The model under review builds one solid part; all positions refer to its coordinate system, in mm. Face numbers are marked on the shaded views. A direction names the side the tool comes from. Round coordinates to 2 decimals unless told otherwise and drop trailing zeros. Order: outer loops, then holes, each group sorted by start corner. A loop starts at its lowest first (then second) coordinate and runs counter-clockwise, first axis right, second up.
```python
from build123d import *

# Parameters (mm, degrees)
PALMA_DEPTH   = 22
MENIQUE_DEPTH = 16
ANULAR_DEPTH  = 16
MEDIO_DEPTH   = 16
INDICE_DEPTH  = 16
PULGAR_DEPTH  = 16


with BuildPart() as part:
    # Sketch1 → Palma (new body)
    with BuildSketch(Plane.XY.offset(-11)):
        Polygon((-36, -27), (36, -27), (40, -60), (38, -118), (-38, -118), (-40, -60), align=None)
    extrude(amount=PALMA_DEPTH)

    # Sketch2 → Menique (add)
    with BuildSketch(Plane.XY.offset(-8)):
        with BuildLine():
            Line((-20.25, -112), (-20.25, -178))
            ThreePointArc((-20.25, -178), (-28.5, -186.25), (-36.75, -178))
            Line((-36.75, -178), (-36.75, -112))
            ThreePointArc((-36.75, -112), (-28.5, -103.75), (-20.25, -112))
        make_face()
    extrude(amount=MENIQUE_DEPTH)

    # Sketch3 → Anular (add)
    with BuildSketch(Plane.XY.offset(-8)):
        with BuildLine():
            Line((-1.25, -112), (-1.25, -194))
            ThreePointArc((-1.25, -194), (-9.5, -202.25), (-17.75, -194))
            Line((-17.75, -194), (-17.75, -112))
            ThreePointArc((-17.75, -112), (-9.5, -103.75), (-1.25, -112))
        make_face()
    extrude(amount=ANULAR_DEPTH)

    # Sketch4 → Medio (add)
    with BuildSketch(Plane.XY.offset(-8)):
        with BuildLine():
            Line((17.75, -112), (17.75, -202))
            ThreePointArc((17.75, -202), (9.5, -210.25), (1.25, -202))
            Line((1.25, -202), (1.25, -112))
            ThreePointArc((1.25, -112), (9.5, -103.75), (17.75, -112))
        make_face()
    extrude(amount=MEDIO_DEPTH)

    # Sketch5 → Indice (add)
    with BuildSketch(Plane.XY.offset(-8)):
        with BuildLine():
            Line((36.75, -112), (36.75, -192))
            ThreePointArc((36.75, -192), (28.5, -200.25), (20.25, -192))
            Line((20.25, -192), (20.25, -112))
            ThreePointArc((20.25, -112), (28.5, -103.75), (36.75, -112))
        make_face()
    extrude(amount=INDICE_DEPTH)

    # Sketch6 → Pulgar (add)
    with BuildSketch(Plane.XY.offset(-13)):
        with BuildLine():
            Line((43.373087285, -56.838838901), (71.373087285, -96.838838901))
            ThreePointArc((71.373087285, -96.838838901), (69.161161099, -109.373087285), (56.626912715, -107.161161099))
            Line((56.626912715, -107.161161099), (28.626912715, -67.161161099))
            ThreePointArc((28.626912715, -67.161161099), (30.838838901, -54.626912715), (43.373087285, -56.838838901))
        make_face()
    extrude(amount=PULGAR_DEPTH)


solid = part.part
```
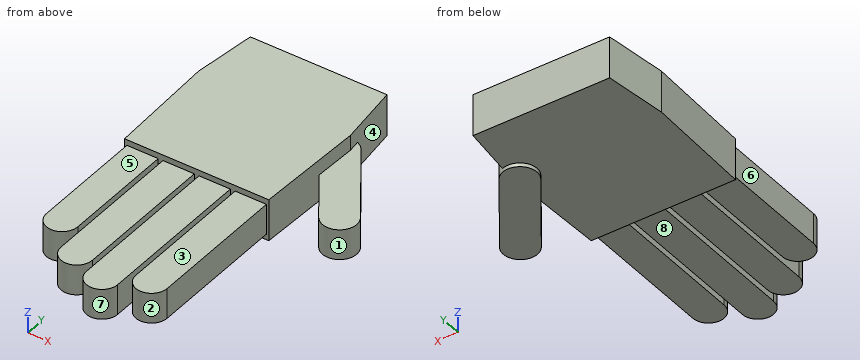
(1) Draft analysis for pull direction X (two halves, no side actions). For the marked faces 1, 2, 3 and 4, state which applies: pulls with the +X half, pulls with the -X half, needs draft (parallel to the pull), parting line crosses it, or undercut.
Data:
face 1: undercut
face 2: undercut
face 3: needs draft
face 4: pulls with the +X half
(2) For the marked faces 5, 6, 7 and 8, list the 3-axis set-ups (+Z, -Z, +X, -X, +Y, -Y) from which the entire face can be reached by the end or side of a thin tool; tool diameter is ignored.
Data:
face 5: +Z, +X, -X, -Y
face 6: +Z, -Z, -X, -Y
face 7: +Z, -Z, -Y
face 8: -Z, +X, -X, -Y
(3) Consider section D-D (z = -5.75). Write out the cut boundary in (x, y).
Data:
outline: (-40, -60) - (-38, -118) - (-36.75, -118) - (-36.75, -178) arc R8.25 ccw to (-20.25, -178) - (-20.25, -118) - (-17.75, -118) - (-17.75, -194) arc R8.25 ccw to (-1.25, -194) - (-1.25, -118) - (1.25, -118) - (1.25, -202) arc R8.25 ccw to (17.75, -202) - (17.75, -118) - (20.25, -118) - (20.25, -192) arc R8.25 ccw to (36.75, -192) - (36.75, -118) - (38, -118) - (39.23, -82.31) - (56.63, -107.16) arc R9 ccw to (71.37, -96.84) - (43.37, -56.84) arc R9 ccw to (39.22, -53.6) - (36, -27) - (-36, -27) - close
(4) Consider section C-C (y = -102). Write out the cut boundary in (x, z).
Data:
outline: (-38.55, -11) - (38.55, -11) - (38.55, 11) - (-38.55, 11) - close; (53.01, -13) - (73, -13) - (73, 3) - (53.01, 3) - close
(5) Consider section A-A (y = -173.5). Write out the cut boundary in (x, z), and give its area (3 significant figures).
Data:
outline: (-36.75, -8) - (-20.25, -8) - (-20.25, 8) - (-36.75, 8) - close; (-17.75, -8) - (-1.25, -8) - (-1.25, 8) - (-17.75, 8) - close; (1.25, -8) - (17.75, -8) - (17.75, 8) - (1.25, 8) - close; (20.25, -8) - (36.75, -8) - (36.75, 8) - (20.25, 8) - close
area: 1,060 mm2
(6) To check wall thickness, follow probe 1 along X at (y, z) = (-134.5, -6); probe 2 along X at (y, z) = (-197, -3.75); probe 3 along Y at (x, z) = (1, -0.5). State the ranges of each line that lie inside material, in increasing order.
Data:
probe 1: x = -36.75 to -20.25, -17.75 to -1.25, 1.25 to 17.75, 20.25 to 36.75
probe 2: x = -17.19 to -1.81, 1.25 to 17.75, 21.94 to 35.06
probe 3: y = -118 to -27
(7) Consider section B-B (x = -28.5). Write out the cut boundary in (y, z), and give its area (3 significant figures).
Data:
outline: (-186.25, -8) - (-118, -8) - (-118, -11) - (-27, -11) - (-27, 11) - (-118, 11) - (-118, 8) - (-186.25, 8) - close
area: 3,090 mm2
(8) Insertion check: pin 1 (5 mm diameter, centred on x = 11, y = -141.5, fed in from -Z); pin 2 (18 mm diameter, centred on x = 30.5, y = -156.5, fed in from +Z); pin 3 (13 mm diameter, centred on y = -168.5, z = -4, fed in from +X). Each pin has a flat end and moves straight along its axis. Give the tip position at first contact, or say it passes through.
Data:
pin 1: stops at z = -8
pin 2: stops at z = 8
pin 3: stops at x = 36.75
